from build123d import *

# Parameters (mm, degrees)
PLATE_FEATURE_DEPTH        = 5
STRAP_FEATURE_SKETCH_RX    = 20
STRAP_FEATURE_SKETCH_RY    = 8
STRAP_FEATURE_DEPTH        = 5
STRAP_CUT_SKETCH_W         = 30
STRAP_CUT_SKETCH_H         = 3.19824666
STRAP_CUT_DEPTH            = 5
LEFT_LEG_FEATURE_SKETCH_W  = 16
LEFT_LEG_FEATURE_SKETCH_H  = 8
LEFT_LEG_FEATURE_DEPTH     = 20
RIGHT_LEG_FEATURE_SKETCH_W = 16
RIGHT_LEG_FEATURE_SKETCH_H = 8
RIGHT_LEG_FEATURE_DEPTH    = 20
TAB_CUT_SKETCH_W           = 8
TAB_CUT_SKETCH_H           = 15
TAB_CUT_DEPTH              = 5
FILLET1_R                  = 10
FILLET2_R                  = 10
FILLET3_R                  = 10


with BuildPart() as part:
    # Plate Feature Sketch → Plate Feature (new body)
    with BuildSketch(Plane.XY):
        Polygon((-36, 18), (-36, 0), (-15.55368079, -50), (18.44631921, -50), (38, 0), (38, 18), align=None)
    extrude(amount=PLATE_FEATURE_DEPTH)

    # Strap Feature Sketch → Strap Feature (add)
    with BuildSketch(Plane.XY):
        with Locations((1.5, -50)):
            Ellipse(STRAP_FEATURE_SKETCH_RX, STRAP_FEATURE_SKETCH_RY)
    extrude(amount=STRAP_FEATURE_DEPTH)

    # Strap Cut Sketch → Strap Cut (cut)
    with BuildSketch(Plane.XY):
        with Locations((1.5, -50.5)):
            Rectangle(STRAP_CUT_SKETCH_W, STRAP_CUT_SKETCH_H)
    extrude(amount=STRAP_CUT_DEPTH, mode=Mode.SUBTRACT)

    # Left Leg Feature Sketch → Left Leg Feature (add)
    with BuildSketch(Plane.XY):
        with Locations((30, 14)):
            Rectangle(LEFT_LEG_FEATURE_SKETCH_W, LEFT_LEG_FEATURE_SKETCH_H)
    extrude(amount=-LEFT_LEG_FEATURE_DEPTH)

    # Right Leg Feature Sketch → Right Leg Feature (add)
    with BuildSketch(Plane.XY):
        with Locations((-28, 14)):
            Rectangle(RIGHT_LEG_FEATURE_SKETCH_W, RIGHT_LEG_FEATURE_SKETCH_H)
    extrude(amount=-RIGHT_LEG_FEATURE_DEPTH)

    # Tab Cut Sketch → Tab Cut (cut)
    with BuildSketch(Plane(origin=(0, 10, 0), x_dir=(1, 0, 0), z_dir=(0, 1, 0))):
        with Locations((-28, 12.5)):
            Rectangle(TAB_CUT_SKETCH_W, TAB_CUT_SKETCH_H)
        with Locations((30, 12.5)):
            Rectangle(TAB_CUT_SKETCH_W, TAB_CUT_SKETCH_H)
    extrude(amount=TAB_CUT_DEPTH, mode=Mode.SUBTRACT)

    # Fillet1
    # the kernel refuses this fillet: 10 mm, written as the material it takes off along each edge
    with BuildSketch(Plane(origin=(63, 18, 5), x_dir=(0, 0, -1), z_dir=(-1, 0, 0))) as fillet1_piece_1:
        with BuildLine():
            CenterArc((FILLET1_R, FILLET1_R), FILLET1_R, 180, 90)
            Line((0, FILLET1_R), (0, 0))
            Line((0, 0), (FILLET1_R, 0))
        make_face()
    extrude(amount=124, mode=Mode.SUBTRACT)

    # Fillet2
    # the kernel refuses this fillet: 10 mm, written as the material it adds along each edge
    with BuildSketch(Plane(origin=(-36, 10, 0), x_dir=(0, 0, -1), z_dir=(1, 0, 0))) as fillet2_piece_1_section:
        with BuildLine():
            CenterArc((FILLET2_R, -FILLET2_R), FILLET2_R, 90, 90)
            Line((0, -FILLET2_R), (0, 0))
            Line((0, 0), (FILLET2_R, 0))
        make_face()
    fillet2_piece_1 = extrude(amount=16, mode=Mode.PRIVATE)
    fillet2_piece_1 = split(fillet2_piece_1, bisect_by=Plane(origin=(-34, 9.759916183, -5), z_dir=(0, 0, -1)), keep=Keep.TOP, mode=Mode.PRIVATE)
    fillet2_piece_1 = split(fillet2_piece_1, bisect_by=Plane(origin=(-32, 9.759916183, -6.632507845), z_dir=(-1, 0, 0)), keep=Keep.TOP, mode=Mode.PRIVATE)
    add(fillet2_piece_1)
    with BuildSketch(Plane(origin=(-36, 10, 0), x_dir=(0, 0, -1), z_dir=(1, 0, 0))) as fillet2_piece_2_section:
        with BuildLine():
            CenterArc((FILLET2_R, -FILLET2_R), FILLET2_R, 90, 90)
            Line((0, -FILLET2_R), (0, 0))
            Line((0, 0), (FILLET2_R, 0))
        make_face()
    fillet2_piece_2 = extrude(amount=16, mode=Mode.PRIVATE)
    fillet2_piece_2 = split(fillet2_piece_2, bisect_by=Plane(origin=(-34, 7.4487994, -5), z_dir=(0, 0, 1)), keep=Keep.TOP, mode=Mode.PRIVATE)
    fillet2_piece_2 = split(fillet2_piece_2, bisect_by=Plane(origin=(-32, 7.4487994, -1.643917643), z_dir=(-1, 0, 0)), keep=Keep.TOP, mode=Mode.PRIVATE)
    add(fillet2_piece_2)
    with BuildSketch(Plane(origin=(-36, 10, 0), x_dir=(0, 0, -1), z_dir=(1, 0, 0))) as fillet2_piece_3_section:
        with BuildLine():
            CenterArc((FILLET2_R, -FILLET2_R), FILLET2_R, 90, 90)
            Line((0, -FILLET2_R), (0, 0))
            Line((0, 0), (FILLET2_R, 0))
        make_face()
    fillet2_piece_3 = extrude(amount=16, mode=Mode.PRIVATE)
    fillet2_piece_3 = split(fillet2_piece_3, bisect_by=Plane(origin=(-24, 7.4487994, -1.643917643), z_dir=(-1, 0, 0)), keep=Keep.TOP, mode=Mode.PRIVATE)
    fillet2_piece_3 = split(fillet2_piece_3, bisect_by=Plane(origin=(-28, 7.4487994, -5), z_dir=(0, 0, 1)), keep=Keep.TOP, mode=Mode.PRIVATE)
    fillet2_piece_3 = split(fillet2_piece_3, bisect_by=Plane(origin=(-32, 7.4487994, -1.643917643), z_dir=(1, 0, 0)), keep=Keep.TOP, mode=Mode.PRIVATE)
    add(fillet2_piece_3)
    with BuildSketch(Plane(origin=(-36, 10, 0), x_dir=(0, 0, -1), z_dir=(1, 0, 0))) as fillet2_piece_4_section:
        with BuildLine():
            CenterArc((FILLET2_R, -FILLET2_R), FILLET2_R, 90, 90)
            Line((0, -FILLET2_R), (0, 0))
            Line((0, 0), (FILLET2_R, 0))
        make_face()
    fillet2_piece_4 = extrude(amount=16, mode=Mode.PRIVATE)
    fillet2_piece_4 = split(fillet2_piece_4, bisect_by=Plane(origin=(-24, 9.759916183, -6.632507845), z_dir=(1, 0, 0)), keep=Keep.TOP, mode=Mode.PRIVATE)
    fillet2_piece_4 = split(fillet2_piece_4, bisect_by=Plane(origin=(-22, 9.759916183, -5), z_dir=(0, 0, -1)), keep=Keep.TOP, mode=Mode.PRIVATE)
    add(fillet2_piece_4)
    with BuildSketch(Plane(origin=(-36, 10, 0), x_dir=(0, 0, -1), z_dir=(1, 0, 0))) as fillet2_piece_5_section:
        with BuildLine():
            CenterArc((FILLET2_R, -FILLET2_R), FILLET2_R, 90, 90)
            Line((0, -FILLET2_R), (0, 0))
            Line((0, 0), (FILLET2_R, 0))
        make_face()
    fillet2_piece_5 = extrude(amount=16, mode=Mode.PRIVATE)
    fillet2_piece_5 = split(fillet2_piece_5, bisect_by=Plane(origin=(-24, 7.4487994, -1.643917643), z_dir=(1, 0, 0)), keep=Keep.TOP, mode=Mode.PRIVATE)
    fillet2_piece_5 = split(fillet2_piece_5, bisect_by=Plane(origin=(-22, 7.4487994, -5), z_dir=(0, 0, 1)), keep=Keep.TOP, mode=Mode.PRIVATE)
    add(fillet2_piece_5)

    # Fillet3
    # the kernel refuses this fillet: 10 mm, written as the material it adds along each edge
    with BuildSketch(Plane(origin=(38, 10, 0), x_dir=(0, 0, -1), z_dir=(-1, 0, 0))) as fillet3_piece_1_section:
        with BuildLine():
            CenterArc((FILLET3_R, FILLET3_R), FILLET3_R, 180, 90)
            Line((0, FILLET3_R), (0, 0))
            Line((0, 0), (FILLET3_R, 0))
        make_face()
    fillet3_piece_1 = extrude(amount=16, mode=Mode.PRIVATE)
    fillet3_piece_1 = split(fillet3_piece_1, bisect_by=Plane(origin=(36, 9.759916183, -5), z_dir=(0, 0, -1)), keep=Keep.TOP, mode=Mode.PRIVATE)
    fillet3_piece_1 = split(fillet3_piece_1, bisect_by=Plane(origin=(34, 9.759916183, -6.632507845), z_dir=(1, 0, 0)), keep=Keep.TOP, mode=Mode.PRIVATE)
    add(fillet3_piece_1)
    with BuildSketch(Plane(origin=(38, 10, 0), x_dir=(0, 0, -1), z_dir=(-1, 0, 0))) as fillet3_piece_2_section:
        with BuildLine():
            CenterArc((FILLET3_R, FILLET3_R), FILLET3_R, 180, 90)
            Line((0, FILLET3_R), (0, 0))
            Line((0, 0), (FILLET3_R, 0))
        make_face()
    fillet3_piece_2 = extrude(amount=16, mode=Mode.PRIVATE)
    fillet3_piece_2 = split(fillet3_piece_2, bisect_by=Plane(origin=(36, 7.4487994, -5), z_dir=(0, 0, 1)), keep=Keep.TOP, mode=Mode.PRIVATE)
    fillet3_piece_2 = split(fillet3_piece_2, bisect_by=Plane(origin=(34, 7.4487994, -1.643917643), z_dir=(1, 0, 0)), keep=Keep.TOP, mode=Mode.PRIVATE)
    add(fillet3_piece_2)
    with BuildSketch(Plane(origin=(38, 10, 0), x_dir=(0, 0, -1), z_dir=(-1, 0, 0))) as fillet3_piece_3_section:
        with BuildLine():
            CenterArc((FILLET3_R, FILLET3_R), FILLET3_R, 180, 90)
            Line((0, FILLET3_R), (0, 0))
            Line((0, 0), (FILLET3_R, 0))
        make_face()
    fillet3_piece_3 = extrude(amount=16, mode=Mode.PRIVATE)
    fillet3_piece_3 = split(fillet3_piece_3, bisect_by=Plane(origin=(26, 7.4487994, -1.643917643), z_dir=(1, 0, 0)), keep=Keep.TOP, mode=Mode.PRIVATE)
    fillet3_piece_3 = split(fillet3_piece_3, bisect_by=Plane(origin=(30, 7.4487994, -5), z_dir=(0, 0, 1)), keep=Keep.TOP, mode=Mode.PRIVATE)
    fillet3_piece_3 = split(fillet3_piece_3, bisect_by=Plane(origin=(34, 7.4487994, -1.643917643), z_dir=(-1, 0, 0)), keep=Keep.TOP, mode=Mode.PRIVATE)
    add(fillet3_piece_3)
    with BuildSketch(Plane(origin=(38, 10, 0), x_dir=(0, 0, -1), z_dir=(-1, 0, 0))) as fillet3_piece_4_section:
        with BuildLine():
            CenterArc((FILLET3_R, FILLET3_R), FILLET3_R, 180, 90)
            Line((0, FILLET3_R), (0, 0))
            Line((0, 0), (FILLET3_R, 0))
        make_face()
    fillet3_piece_4 = extrude(amount=16, mode=Mode.PRIVATE)
    fillet3_piece_4 = split(fillet3_piece_4, bisect_by=Plane(origin=(26, 9.759916183, -6.632507845), z_dir=(-1, 0, 0)), keep=Keep.TOP, mode=Mode.PRIVATE)
    fillet3_piece_4 = split(fillet3_piece_4, bisect_by=Plane(origin=(24, 9.759916183, -5), z_dir=(0, 0, -1)), keep=Keep.TOP, mode=Mode.PRIVATE)
    add(fillet3_piece_4)
    with BuildSketch(Plane(origin=(38, 10, 0), x_dir=(0, 0, -1), z_dir=(-1, 0, 0))) as fillet3_piece_5_section:
        with BuildLine():
            CenterArc((FILLET3_R, FILLET3_R), FILLET3_R, 180, 90)
            Line((0, FILLET3_R), (0, 0))
            Line((0, 0), (FILLET3_R, 0))
        make_face()
    fillet3_piece_5 = extrude(amount=16, mode=Mode.PRIVATE)
    fillet3_piece_5 = split(fillet3_piece_5, bisect_by=Plane(origin=(26, 7.4487994, -1.643917643), z_dir=(-1, 0, 0)), keep=Keep.TOP, mode=Mode.PRIVATE)
    fillet3_piece_5 = split(fillet3_piece_5, bisect_by=Plane(origin=(24, 7.4487994, -5), z_dir=(0, 0, 1)), keep=Keep.TOP, mode=Mode.PRIVATE)
    add(fillet3_piece_5)


solid = part.part
Input: part model. Units: mm. Frame: model coordinates. A direction names the side the tool comes from. Coordinates: 2 decimals unless noted, no trailing zeros. Loops run counter-clockwise (first coordinate to the right, second up) from the corner with the lowest first, then second, coordinate; pieces in that order, holes last. Notation, with made-up numbers: (-40, 89) -> (-4, 89) arc R15 cw to (-4, 100) -> close; hole circle Ø2 at (83.5, 3.25). An arc over 180 degrees is marked (long way). Write each question's results on one line, items separated by ' | '. Start each with the question number.
Q1. Section C-C, the plane x = -23. Return the cut outline in (y, z), plus the area to 3 significant figures.
Q2. Reachability of faces 4 (the flat face through (22, 13, -10)), 5 (the flat face through (1, -48.901, 2)), 6 (the flat face through (36, 10, -15)), 7 (the flat face through (34, 12, -13)) from +Z, -Z, +X, -X, +Y, -Y: full face, straight path, thin tool, end or side. Return the list, or none.
Q3. Section D-D, the plane z = -7.5. Return the cut outline in (x, y).
Q4. Ray query, line 1 (X direction, y = 13, z = -6.5); line 2 (X direction, y = 10, z = -2); line 3 (Z direction, x = 2.5, y = -7). Return the intervals inside material, ascending. Write a range as from..to.
Q5. Pin query (flat end, axial travel): pin 1 (1 mm diameter, centred on y = -51, z = 2, fed in from +X); pin 2 (3 mm diameter, centred on x = -22, z = -12.5, fed in from -Y); pin 3 (10 mm diameter, centred on x = -24.5, y = -6, fed in from -Z). Return the tip coordinate at first contact, or that it passes through.
Q6. Section B-B, the plane y = 6.5. Return the cut outline in (x, z).
Q7. Pull-direction query (Y, two-part tool) for faces 1 (the flat face through (30, 12, -5)), 2 (the flat face through (30, 18, -12)), 3 (the flat face through (-13.5, -51, 2)); classes: released by +Y, released by -Y, zero draft, split by the parting line, or undercut.
Q8. Section A-A, the plane z = -15.75. Return the cut outline in (x, y), plus the area to 3 significant figures.
Found:
1) outline: (-31.79, 0) -> (0, 0) arc R10 cw to (10, -10) -> (10, -20) -> (18, -20) -> (18, -5) arc R10 ccw to (8, 5) -> (-31.79, 5) -> close | area: 409 mm2
2) face 4: -Z, +Y, -Y | face 5: +Z, -Z | face 6: -Z, +X, -X, -Y | face 7: -Z, -Y
3) outline: (-36, 9.68) -> (-32, 9.68) -> (-32, 15) -> (-24, 15) -> (-24, 9.68) -> (-20, 9.68) -> (-20, 18) -> (-36, 18) -> close; (22, 9.68) -> (26, 9.68) -> (26, 15) -> (34, 15) -> (34, 9.68) -> (38, 9.68) -> (38, 18) -> (22, 18) -> close
4) line 1: -36..-32, -24..-20, 22..26, 34..38 | line 2: -36..-20, 22..38 | line 3: 0..5
5) pin 1: x = 21.46 | pin 2: y = 10 | pin 3: z = 0
6) outline: (-36, -2.4) -> (-20, -2.4) -> (-20, 0) -> (22, 0) -> (22, -2.4) -> (38, -2.4) -> (38, 5) -> (-36, 5) -> close
7) face 1: zero draft | face 2: released by +Y | face 3: undercut
8) outline: (-36, 10) -> (-32, 10) -> (-32, 15) -> (-24, 15) -> (-24, 10) -> (-20, 10) -> (-20, 18) -> (-36, 18) -> close; (22, 10) -> (26, 10) -> (26, 15) -> (34, 15) -> (34, 10) -> (38, 10) -> (38, 18) -> (22, 18) -> close | area: 176 mm2
